from build123d import *

# Parameters (mm, degrees)
F1_DEPTH = 63.5
F2_DEPTH = 25.4
F3_DEPTH = 12.7
F0_W     = 40.8507403036
F0_H     = 38.1
F5_R     = 5.08


with BuildPart() as f1:
    # F0 (on Front) → F1 (new body, symmetric)
    with BuildSketch(Plane.XZ):
        Polygon((44.45, -14.2875), (44.45, 14.2875), (27.6001971215, 14.2875), (-44.45, 14.2875), (-44.45, -14.2875), align=None)
    extrude(amount=F1_DEPTH, both=True)

    # F0 (on Front) → F2 (join, symmetric)
    with BuildSketch(Plane.XZ):
        with BuildLine():
            Line((27.6001971215, 14.2875), (44.45, 14.2875))
            Line((44.45, 14.2875), (44.45, 58.7375))
            ThreePointArc((44.45, 58.7375), (49.0996798487, 69.9628201513), (60.325, 74.6125))
            Line((60.325, 74.6125), (66.6749985714, 74.6125))
            Line((66.6749985714, 74.6125), (66.6749985714, 91.4623028785))
            Line((66.6749985714, 91.4623028785), (60.325, 91.4623028785))
            ThreePointArc((60.325, 91.4623028785), (37.1850699716, 81.8774300284), (27.6001971215, 58.7375))
            Line((27.6001971215, 58.7375), (27.6001971215, 14.2875))
        make_face()
        Polygon((66.6749985714, 91.4623028785), (66.6749985714, 74.6125), (66.6749985714, 61.9125), (89.3242582679, 61.9125), (89.3242582679, 100.0125), (66.6749985714, 100.0125), align=None)
    extrude(amount=F2_DEPTH, both=True)

    # F0 (on Front) → F3 (join, symmetric)
    with BuildSketch(Plane.XZ):
        with BuildLine():
            Line((-44.45, 14.2875), (27.6001971215, 14.2875))
            Line((27.6001971215, 14.2875), (27.6001971215, 58.7375))
            ThreePointArc((27.6001971215, 58.7375), (37.1850699716, 81.8774300284), (60.325, 91.4623028785))
            add(Edge.make_bspline(
                [(-44.45, 14.2875), (-23.5856175423, 54.6985641122), (19.0692264587, 93.3388397098), (60.325, 91.4623028785)],
                knots=[0, 0, 0, 0, 130.1297461165, 130.1297461165, 130.1297461165, 130.1297461165], degree=3))
        make_face()
    extrude(amount=F3_DEPTH, both=True)

    # F0 (on Front) → F4 (revolve)
    with BuildSketch(Plane.XZ):
        with Locations((109.7496284197, 80.9625)):
            Rectangle(F0_W, F0_H)
    revolve(axis=Axis((89.3242582679, 0, 80.9625), (0, 0, 1)))

    # F5
    f5_edges = [f1.edges().sort_by_distance(p)[0] for p in [
        (44.45, -63.5, 0),
        (-44.45, -63.5, 0),
        (44.45, 63.5, 0),
        (-44.45, 63.5, 0),
    ]]
    fillet(f5_edges, radius=F5_R)


solid = f1.part
The listing builds one solid part. Answer for the finished solid, in the listing's coordinates (mm). A direction names the side the tool comes from. Give positions to 0.01 mm unless a question says otherwise; leave off trailing zeros. Write each loop counter-clockwise with the first axis right and the second up, starting at its lowest first coordinate (ties: lowest second). Pieces come first, ordered by that corner, then holes.
Item 1: Determine the mould class of faces 5 (the cylindrical face through (36.379, -19.139, 81.042)), 6 (the flat face through (2, 12.7, 45)), 7 (the flat face through (-1, -1, -14.288)) for opening direction Z: released by +Z, released by -Z, zero draft, split by the parting line, or undercut.
Item 2: Find the intervals of material crossed by line 1 along Z through (x, y) = (55, -6); line 2 along Z through (x, y) = (-31.5, 28); line 3 along Y through (x, z) = (21, 50.5), in increasing order.
Item 3: Section A-A, the plane z = 12 is taken. Write down the section's boundary in (x, y).
Item 4: Section B-B, the plane x = 108.5 is taken. Write down the section's boundary in (y, z), plus the area to 3 significant figures.
Item 5: Flat-ended cylindrical pins translate along their axes: P1, Ø10, axis at y = 18, z = 40.5, coming from the -X side; P2, Ø14, axis at y = -19, z = 44, coming from the -X side; P3, Ø4, axis at x = 5, y = -23, coming from the +Z side. Find the tip coordinate at first contact, or state that the pin passes through.
Item 6: Which of the six approach directions +Z, -Z, +X, -X, +Y, -Y give full straight-line access (tool end or side, diameter ignored) to faces 1 (the flat face through (90, 1, 61.913)), 2 (the flat face through (-1, 63.5, 0)), 3 (the flat face through (1, -38, 14.288)), 4 (the flat face through (1, 38, 14.288))?
Completed:
1. face 5: released by +Z
1. face 6: zero draft
1. face 7: released by -Z
2. line 1: z = 61.91 to 100.01
2. line 2: z = -14.29 to 14.29
2. line 3: y = -12.7 to 12.7
3. outline: (-44.45, -58.42) arc R5.08 ccw to (-39.37, -63.5) - (39.37, -63.5) arc R5.08 ccw to (44.45, -58.42) - (44.45, 58.42) arc R5.08 ccw to (39.37, 63.5) - (-39.37, 63.5) arc R5.08 ccw to (-44.45, 58.42) - close
4. outline: (-36.07, 61.91) - (36.07, 61.91) - (36.07, 100.01) - (-36.07, 100.01) - close
4. area: 2,750 mm2
5. P1: stops at x = 27.6
5. P2: stops at x = -27.25
5. P3: stops at z = 14.29
6. face 1: -Z, +X, +Y, -Y
6. face 2: +Z, -Z, +X, -X, +Y
6. face 3: +Z, -X, -Y
6. face 4: +Z, -X, +Y
